```python
from build123d import *

# Parameters (mm, degrees)
F1_DEPTH = 4
F2_D     = 3.4


with BuildPart() as f1:
    # F0 (on Front) → F1 (new body)
    with BuildSketch(Plane.XZ):
        with BuildLine():
            Line((60, 5), (0, 5))
            ThreePointArc((0, 5), (-5, 0), (0, -5))
            Line((0, -5), (60, -5))
            ThreePointArc((60, -5), (65, 0), (60, 5))
        make_face()
    extrude(amount=F1_DEPTH)

    # F2 (through all)
    with Locations(Plane(origin=(0, 0, 0), x_dir=(1, 0, 0), z_dir=(0, 1, 0))):
        with Locations((0, 0), (60, 0)):
            Hole(F2_D / 2)


solid = f1.part
```
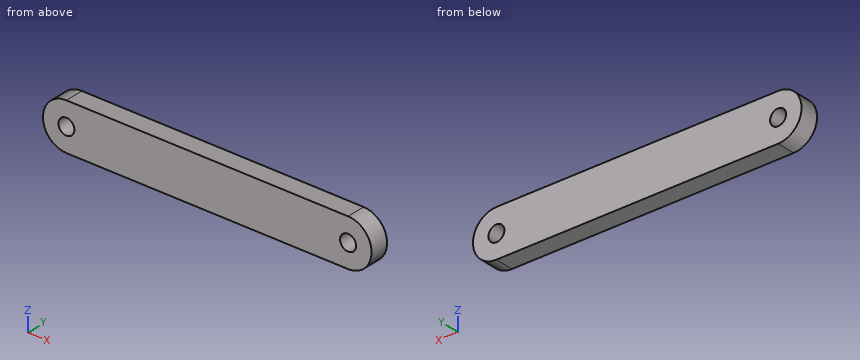
Input: part model. Units: mm. Frame: model coordinates. Give positions to 0.01 mm unless a question says otherwise; leave off trailing zeros. Order: outer loops, then holes, each group sorted by start corner. A loop starts at its lowest first (then second) coordinate and runs counter-clockwise, first axis right, second up.
1. Section C-C on z = -3. Return the cut outline in (x, y), and give its area (3 significant figures).
Derived:
outline: (-4, -4) - (64, -4) - (64, 0) - (-4, 0) - close
area: 272 mm2
2. Material intervals for L1, parallel to X at y = -1, z = 0.75; L2, parallel to X at y = -3.25, z = 1.25; L3, parallel to Z at x = 0, y = -2.4, sorted ascending.
Derived:
L1: x = -4.94 to -1.53, 1.53 to 58.47, 61.53 to 64.94
L2: x = -4.84 to -1.15, 1.15 to 58.85, 61.15 to 64.84
L3: z = -5 to -1.7, 1.7 to 5
3. Pin query (flat end, axial travel): pin 1 (3 mm diameter, centred on x = 0, z = 0, fed in from +Y). Return the tip coordinate at first contact, or that it passes through.
Derived:
pin 1: passes through
4. Section D-D on z = 3.5. Return the cut outline in (x, y).
Derived:
outline: (-3.57, -4) - (63.57, -4) - (63.57, 0) - (-3.57, 0) - close
5. Section B-B on y = -1.3. Return the cut outline in (x, z), and give its area (3 significant figures).
Derived:
outline: (0, -5) - (60, -5) arc R5 ccw to (60, 5) - (0, 5) arc R5 ccw to start; hole circle Ø3.4 at (0, 0); hole circle Ø3.4 at (60, 0)
area: 660 mm2
6. Section A-A on z = 0. Return the cut outline in (x, y), and give its area (3 significant figures).
Derived:
outline: (-5, -4) - (-1.7, -4) - (-1.7, 0) - (-5, 0) - close; (1.7, -4) - (58.3, -4) - (58.3, 0) - (1.7, 0) - close; (61.7, -4) - (65, -4) - (65, 0) - (61.7, 0) - close
area: 253 mm2
